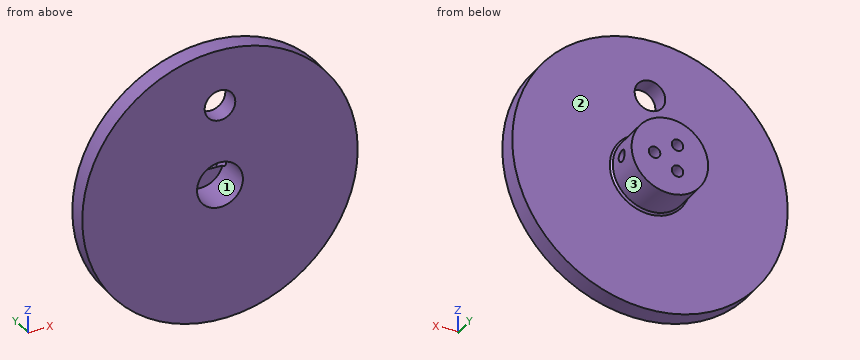
```python
from build123d import *

# Parameters (mm, degrees)
F0_R          = 36
F1_DEPTH      = 15
F2_R          = 65
F2_R_2        = 10
F3_DEPTH      = 10
F4_SIZE       = 0.5
F5_R          = 1.5
F6_DEPTH      = 25
F6_DEPTH_BACK = 25
F7_R          = 4
F8_DEPTH      = 25
F9_R          = 1.5
F10_DEPTH     = 15
F11_R         = 6
F12_DEPTH     = 10


with BuildPart() as f1:
    # F0 (on Front) → F1 (new body)
    with BuildSketch(Plane.XZ):
        Circle(F0_R)
    extrude(amount=F1_DEPTH)

    # F2 (on face) → F3 (cut)
    with BuildSketch(Plane(origin=(0, 0, 0), x_dir=(-1, 0, 0), z_dir=(0, 1, 0))):
        Circle(F2_R)
        Circle(F2_R_2, mode=Mode.SUBTRACT)
    extrude(amount=-F3_DEPTH, mode=Mode.SUBTRACT)

    # F4
    f4_edges = [f1.edges().sort_by_distance(p)[0] for p in [
        (10, -10, 0),
    ]]
    chamfer(f4_edges, length=F4_SIZE)

    # F5 (on Right) → F6 (cut, two sides)
    with BuildSketch(Plane.YZ) as f6_sk:
        with Locations((-5, 0)):
            Circle(F5_R)
    extrude(amount=F6_DEPTH, mode=Mode.SUBTRACT)
    extrude(f6_sk.sketch, amount=-F6_DEPTH_BACK, mode=Mode.SUBTRACT)

    # F7 (on Front) → F8 (cut)
    with BuildSketch(Plane.XZ):
        with Locations((0, 21.25)):
            Circle(F7_R)
    extrude(amount=F8_DEPTH, mode=Mode.SUBTRACT)

    # F9 (on Front) → F10 (cut)
    with BuildSketch(Plane.XZ):
        with Locations((-2, 3.464102)):
            Circle(F9_R)
        with Locations((-2, -3.464102)):
            Circle(F9_R)
        with Locations((4, 0)):
            Circle(F9_R)
    extrude(amount=F10_DEPTH, mode=Mode.SUBTRACT)

    # F11 (on face) → F12 (cut)
    with BuildSketch(Plane.XZ.offset(15)):
        Circle(F11_R)
    extrude(amount=-F12_DEPTH, mode=Mode.SUBTRACT)


solid = f1.part
```
Source: CAD feature listing. Evaluate the final solid. Frame: model axes, mm. Face numbers are marked on the shaded views. Coordinates: 2 decimals unless noted, no trailing zeros. Loops run counter-clockwise (first coordinate to the right, second up) from the corner with the lowest first, then second, coordinate; pieces in that order, holes last. Notation, with made-up numbers: (54.5, 39.5) -> (98.5, 39.5) arc R24 cw to (98.5, 64.5) -> close; hole circle Ø7 at (-12, 84.25). An arc over 180 degrees is marked (long way). One line per item, written item: value. Start each with the question number.
Q1. Section query A-A, the plane z = 0. Return the cut outline in (x, y), and give its area (3 significant figures).
Q2. Contact query for flat-ended pins moving along their axis: P1, Ø15.5, axis at x = 0, z = 0, coming from the -Y side; P2, Ø8, axis at y = -4.5, z = -12.5, coming from the +X side; P3, Ø4, axis at y = -5, z = 0, coming from the +X side; P4, Ø3, axis at x = 26, z = -12, coming from the +Y side. Output: stop coordinate, or through.
Q3. Section query B-B, the plane z = 21.25. Return the cut outline in (x, y).
Q4. Line query: line 1 along X through (y, z) = (-10.5, 0); line 2 along Z through (x, y) = (-2, -3.8); line 3 along X through (y, z) = (-1.95, 0). Output: solid intervals per line, ascending.
Q5. Section query C-C, the plane y = -2. Return the cut outline in (x, z), and give its area (3 significant figures).
Q6. Mould query, pull axis Z, two halves, no side actions, for the marked faces 1, 2 and 3. Classes: pulls with the +Z half, pulls with the -Z half, needs draft (parallel to the pull), parting line crosses it, or undercut.
Q7. Section query D-D, the plane x = -1.5. Give the number of separate pieces and of enclosed holes in the cut face, and give its area (3 significant figures).
Results:
1. outline: (-36, -15) -> (-6, -15) -> (-6, -6.5) -> (-10, -6.5) -> (-10, -9.5) -> (-10.5, -10) -> (-36, -10) -> close; (-10, -3.5) -> (2.5, -3.5) -> (2.5, 0) -> (-10, 0) -> close; (5.5, -3.5) -> (10, -3.5) -> (10, 0) -> (5.5, 0) -> close; (6, -15) -> (36, -15) -> (36, -10) -> (10.5, -10) -> (10, -9.5) -> (10, -6.5) -> (6, -6.5) -> close
1. area: 388 mm^2
2. P1: y = -15
2. P2: x = 5.27
2. P3: x = 10
2. P4: y = -10
3. outline: (-29.06, -15) -> (-4, -15) -> (-4, -10) -> (-29.06, -10) -> close; (4, -15) -> (29.06, -15) -> (29.06, -10) -> (4, -10) -> close
4. line 1: -36 to -6, 6 to 36
4. line 2: -9.8 to -4.96, -1.96 to -0.9, 0.9 to 1.96, 4.96 to 9.8
4. line 3: -10 to 2.5, 5.5 to 10
5. outline: circle Ø20 at (0, 0); hole circle Ø3 at (-2, -3.46); hole circle Ø3 at (-2, 3.46); hole circle Ø3 at (4, 0)
5. area: 293 mm^2
6. face 1: undercut
6. face 2: needs draft
6. face 3: parting line crosses it
7. separate pieces: 4
7. enclosed holes: 0
7. area: 373 mm^2
